```python
from build123d import *

# Parameters (mm, degrees)
CYLINDER076_R                            = 2
CYLINDER076_DEPTH                        = 1
BOX406008005_W                           = 16
BOX406008005_H                           = 10
BOX406008005_DEPTH                       = 27
CYLINDER077_R                            = 6
CYLINDER077_DEPTH                        = 15
BOX406008006_W                           = 10
BOX406008006_H                           = 10
BOX406008006_DEPTH                       = 12
CYLINDER078_R                            = 1.5
CYLINDER078_DEPTH                        = 10
BOX406008004_W                           = 12
BOX406008004_H                           = 10
BOX406008004_DEPTH                       = 9
FUSION103077013004017004_PLACEMENT_ANGLE = 45


with BuildPart() as boss002:
    # Cylinder076 → Cylinder076 (new body)
    with BuildSketch(Plane.XY.offset(-1)):
        Circle(CYLINDER076_R)
    extrude(amount=CYLINDER076_DEPTH)


with BuildPart() as gearbox005:
    # Box406008005 → Box406008005 (new body)
    with BuildSketch(Plane(origin=(-8, -5, 0), x_dir=(1, 0, 0), z_dir=(0, 0, 1))):
        with Locations((8, 5)):
            Rectangle(BOX406008005_W, BOX406008005_H)
    extrude(amount=BOX406008005_DEPTH)


with BuildPart() as motor002:
    # Cylinder077 → Cylinder077 (new body)
    with BuildSketch(Plane.XY.offset(9)):
        Circle(CYLINDER077_R)
    extrude(amount=CYLINDER077_DEPTH)

    # Common001: intersect gearbox005
    add(gearbox005.part, mode=Mode.INTERSECT)


with BuildPart() as cube341:
    # Box406008006 → Box406008006 (new body)
    with BuildSketch(Plane(origin=(-5, 1, -11), x_dir=(1, 0, 0), z_dir=(0, 0, 1))):
        with Locations((5, 5)):
            Rectangle(BOX406008006_W, BOX406008006_H)
    extrude(amount=BOX406008006_DEPTH)


with BuildPart() as shaft002:
    # Cylinder078 → Cylinder078 (new body)
    with BuildSketch(Plane.XY.offset(-10)):
        Circle(CYLINDER078_R)
    extrude(amount=CYLINDER078_DEPTH)

    # Cut001: cut Cube341
    add(cube341.part, mode=Mode.SUBTRACT)


with BuildPart() as motor_assembled:
    # Box406008004 → Box406008004 (new body)
    with BuildSketch(Plane(origin=(-6, -5, 0), x_dir=(1, 0, 0), z_dir=(0, 0, 1))):
        with Locations((6, 5)):
            Rectangle(BOX406008004_W, BOX406008004_H)
    extrude(amount=BOX406008004_DEPTH)

    # Fusion103077013004017004: union boss002, motor002, shaft002
    add(boss002.part)
    add(motor002.part)
    add(shaft002.part)


with BuildPart() as motor_assembled_1:
    # Fusion103077013004017004 placement: moved
    add(motor_assembled.part.moved(Location((0, 0, 20.5))).rotate(Axis((0, 0, 20.5), (0, 0, -1)), FUSION103077013004017004_PLACEMENT_ANGLE))


solid = motor_assembled_1.part
```
Here's how the part is built. I have some questions about the finished solid (model axes, mm). A direction names the side the tool comes from. Give positions to 0.01 mm unless a question says otherwise; leave off trailing zeros. Order: outer loops, then holes, each group sorted by start corner. A loop starts at its lowest first (then second) coordinate and runs counter-clockwise, first axis right, second up. Notation, with made-up numbers: M 79,40.5 L 114,40.5 A17 ccw 114,73.5 Z; hole C 55,11.25 d9. An arc over 180 degrees is marked long. Use a Markdown table: item, result. Add a question column.
1. Suppose I cut it at D-D (z = 38). List the corners of the cut face in (x, y) for me, and give its area (3 significant figures).
2. Suppose I cut it at A-A (x = -5). List the corners of the cut face in (y, z) for me, and give its area (3 significant figures).
3. For pin 1 Ø2 at (y, z) = (1, 18) entering from -X; pin 2 Ø1 at (x, y) = (-4.5, -3) entering from -Z; pin 3 Ø1.5 at (y, z) = (-0.5, 29.5) entering from +X; pin 4 Ø6 at (y, z) = (-3.5, 19) entering from -X, each with a flat end and sliding along its axis, tell me the tip position at first contact or that it passes through.
4. On a 3-axis mill with a long thin cutter (end or side, diameter ignored), from which of +Z, -Z, +X, -X, +Y, -Y can I reach the whole of each face in a straight line? I mean faces 1 (the flat face through (0.696, 0.718, 14.937)), 2 (the flat face through (-4.292, 4.193, 24.937)), 3 (the flat face through (1, 1, 19.5)). Say none if no direction works.
5. If we mould it in two halves opening along X, with no side actions, what happens to faces 4 (the flat face through (1.1, -6.5, 29.5)), 5 (the flat face through (4.193, -4.292, 24.937)), 6 (the cylindrical face through (2, 0, 20))? For each: +X half, -X half, draft (parallel to the pull), parting line (faces both ways), or undercut.
6. I need wall thicknesses on probe 1 along X at (y, z) = (-0.25, 38.5); probe 2 along Z at (x, y) = (4.25, 1.25); probe 3 along Z at (x, y) = (6.25, 0). Which ranges of each line are inside material? Lowest first, please. Write a range as from..to.
7. Suppose I cut it at C-C (z = 22.5). List the corners of the cut face in (x, y) for me, and give its area (3 significant figures).
8. Suppose I cut it at B-B (y = -2.75). List the corners of the cut face in (x, z) for me.
Results list:
| question | item | result |
|---|---|---|
| 1 | outline | M -5.88,-1.19 L -1.19,-5.88 A6 ccw 5.88,1.19 L 1.19,5.88 A6 ccw Z |
| 1 | area | 104 mm² |
| 2 | outline | M -2.07,20.5 L 3.49,20.5 L 3.49,29.5 L 3.32,29.5 L 3.32,44.5 L -2.07,44.5 Z |
| 2 | area | 131 mm² |
| 3 | pin 1 | stops at x = -1.5 |
| 3 | pin 2 | stops at z = 20.5 |
| 3 | pin 3 | stops at x = 7.78 |
| 3 | pin 4 | stops at x = -6.17 |
| 4 | face 1 | -Z, +X, +Y |
| 4 | face 2 | +Z, -Z, -X, +Y |
| 4 | face 3 | -Z |
| 5 | face 4 | draft |
| 5 | face 5 | +X half |
| 5 | face 6 | parting line |
| 6 | probe 1 | x = -5.99..5.99 |
| 6 | probe 2 | z = 20.5..44.5 |
| 6 | probe 3 | z = 20.5..29.5 |
| 7 | outline | M -7.78,0.71 L 0.71,-7.78 L 7.78,-0.71 L -0.71,7.78 Z |
| 7 | area | 120 mm² |
| 8 | outline | M -4.32,20.5 L 5.74,20.5 L 5.74,29.5 L 5.33,29.5 L 5.33,44.5 L -4.32,44.5 Z |
